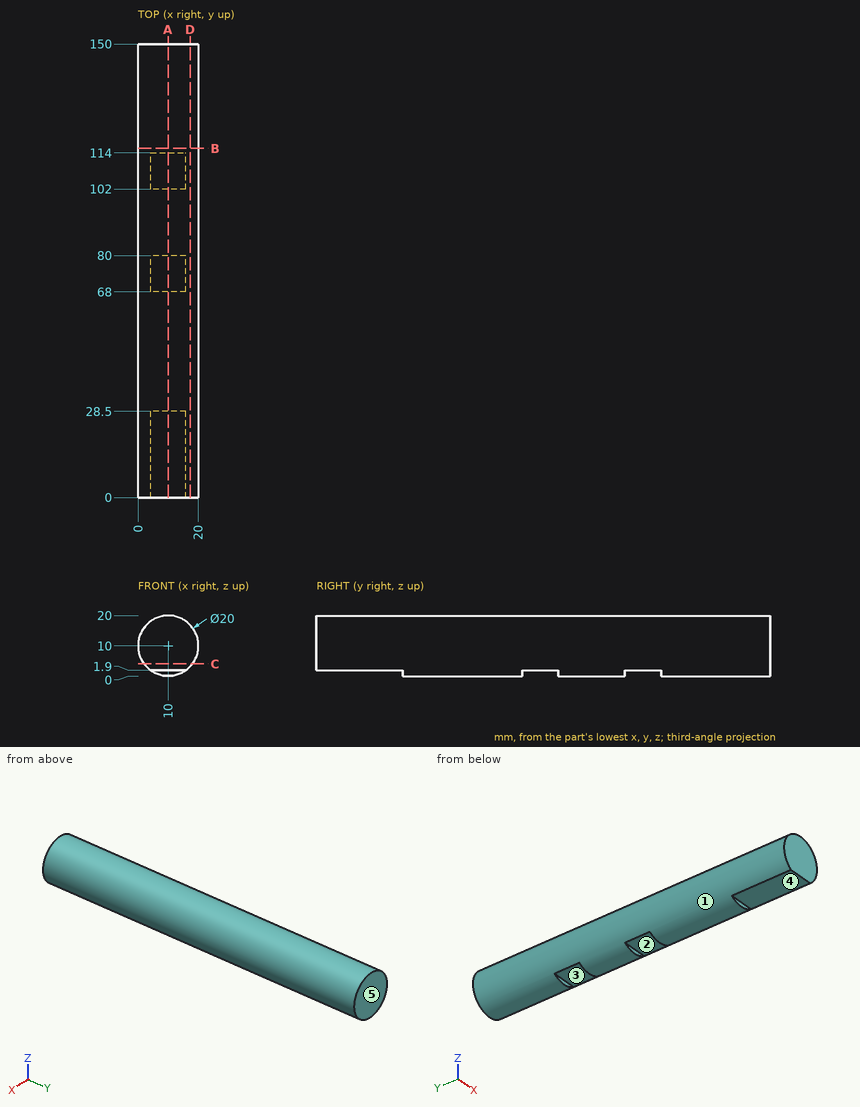
Verification items for this drawing (mm, ordinates from the low corner). A direction names the side the tool comes from. Round coordinates to 2 decimals unless told otherwise and drop trailing zeros. Order: outer loops, then holes, each group sorted by start corner. A loop starts at its lowest first (then second) coordinate and runs counter-clockwise, first axis right, second up. Notation, with made-up numbers: M 22,51 L 74,51 A21 ccw 74,74 Z; hole C 2.25,76 d3. An arc over 180 degrees is marked long. Answer in a Markdown table with one row per item. Add a question column.
Item 1: Sectioned sample at D-D, the plane x = 17.25. Enter the section's corners in (y, z), plus the area to 3 significant figures.
Item 2: Material ranges on L1, parallel to Y at x = 6.75, z = 1; L2, parallel to X at y = 110.5, z = 15; L3, parallel to Z at x = 8.5, y = 59.5, recorded low to high. Write a range as [from, to].
Item 3: Depth check by flat-ended pin: pin 1 Ø4 at (y, z) = (43, 16) entering from +X; pin 2 Ø10 at (y, z) = (87.5, 17) entering from +X; pin 3 Ø1 at (x, z) = (7.5, 1) entering from -Y. Enter the tip coordinate at first touch or a pass-through.
Item 4: Sectioned sample at A-A, the plane x = 10. Enter the section's corners in (y, z).
Item 5: Draft check along Y on the marked faces 3, 4 and 5. Enter one of: released by +Y, released by -Y, zero draft, split by the parting line, or undercut.
Item 6: Set-up check for the marked faces 1 and 2: record each of +Z, -Z, +X, -X, +Y, -Y from which the full face is reachable in a straight line by a thin tool's end or side.
Item 7: Sectioned sample at B-B, the plane y = 115.5. Enter the section's corners in (x, z), plus the area to 3 significant figures.
Item 8: Sectioned sample at C-C, the plane z = 4. Enter the section's corners in (x, y), plus the area to 3 significant figures.
Filled in:
| question | item | result |
|---|---|---|
| 1 | outline | M 0,3.11 L 150,3.11 L 150,16.89 L 0,16.89 Z |
| 1 | area | 2,070 mm² |
| 2 | L1 | y = [28.5, 68], [80, 102], [114, 150] |
| 2 | L2 | x = [1.34, 18.66] |
| 2 | L3 | z = [0.11, 19.89] |
| 3 | pin 1 | stops at x = 19.17 |
| 3 | pin 2 | stops at x = 19.8 |
| 3 | pin 3 | stops at y = 28.5 |
| 4 | outline | M 0,1.9 L 28.5,1.9 L 28.5,0 L 68,0 L 68,1.9 L 80,1.9 L 80,0 L 102,0 L 102,1.9 L 114,1.9 L 114,0 L 150,0 L 150,20 L 0,20 Z |
| 5 | face 3 | undercut |
| 5 | face 4 | zero draft |
| 5 | face 5 | released by +Y |
| 6 | face 1 | +Y, -Y |
| 6 | face 2 | -Z, +X, -X |
| 7 | outline | C 10,10 d20 |
| 7 | area | 314 mm² |
| 8 | outline | M 2,0 L 18,0 L 18,150 L 2,150 Z |
| 8 | area | 2,400 mm² |
